from build123d import *

# Parameters (mm, degrees)
FORO_SVASATO_PER_VITE_M5_1_D           = 5
FORO_SVASATO_PER_VITE_M5_1_CSINK_D     = 8.6
FORO_SVASATO_PER_VITE_M5_1_CSINK_ANGLE = 90
RIPETIZIONECIRCOLARE1_COUNT            = 4


with BuildPart() as part:
    # Schizzo1 → Rivoluzione1 (revolve)
    with BuildSketch(Plane.XY, mode=Mode.PRIVATE) as rivoluzione1_sk:
        Polygon((6.5, 0), (6.5, 4), (9, 4), (9, 9), (23, 9), (23, 4.7), (12.5, 4.7), (12.5, 0), align=None)
    revolve(rivoluzione1_sk.sketch.rotate(Axis((0, 0, 0), (0, 1, 0)), 90), axis=Axis((0, 0, 0), (0, 1, 0)))

    # Foro svasato per Vite M5-1 (through all)
    with Locations(Plane(origin=(0, 4.7, 0), x_dir=(-1, 0, 0), z_dir=(0, -1, 0))):
        with Locations((-17.5, 0)):
            foro_svasato_per_vite_m5_1 = CounterSinkHole(FORO_SVASATO_PER_VITE_M5_1_D / 2, FORO_SVASATO_PER_VITE_M5_1_CSINK_D / 2, counter_sink_angle=FORO_SVASATO_PER_VITE_M5_1_CSINK_ANGLE)

    # RipetizioneCircolare1: Foro svasato per Vite M5-1 ×4 about axis
    ripetizionecircolare1_axis = Axis((0, 0, 0), (0, 1, 0))
    for i in range(1, RIPETIZIONECIRCOLARE1_COUNT):
        add(foro_svasato_per_vite_m5_1.rotate(ripetizionecircolare1_axis, i * 360 / RIPETIZIONECIRCOLARE1_COUNT), mode=Mode.SUBTRACT)


solid = part.part
CAD build for the part. Positions are in the model's coordinates, mm. A direction names the side the tool comes from. Give positions to 0.01 mm unless a question says otherwise; leave off trailing zeros. Loops run counter-clockwise (first coordinate to the right, second up) from the corner with the lowest first, then second, coordinate; pieces in that order, holes last. Notation, with made-up numbers: M 74,83.5 L 103,83.5 A20 ccw 103,100.5 Z; hole C -17.75,-35 d7. An arc over 180 degrees is marked long. One line per question, with ' | ' between items. Start each with the question number.
1. 3-axis set-ups, long thin cutter, end or side, ignore diameter. For faces 1 (the face through (10, 4.7, -10)), 2 (the face through (6, 4, 3)), 3 (the face through (15, 8, 0)): which of +Z, -Z, +X, -X, +Y, -Y reach the whole face in a straight line?
2. Saw through at A-A on x = 0. Give the cut face in (y, z), plus the area to 3 significant figures.
3. Saw through at C-C on y = 5.25. Give the cut face in (x, z).
4. Saw through at D-D on z = 0. Give the cut face in (x, y).
5. Two-plate mould, pull along X, no slides. Class faces 4 (the face through (-3.755, 2.317, -11.923)), 5 (the face through (0, 9, 10)), 6 (the face through (-15, 8, 0)): pulls with the +X half, pulls with the -X half, needs draft (parallel to the pull), parting line crosses it, or undercut.
6. Probe L1, parallel to Z at x = 17.5, y = 7.4; L2, parallel to Y at x = -16.5, z = -14. List the from-to ranges inside material, lowest first. Write a range as from..to.
7. Flat gauge pins, fed straight in: pin 1 (14 mm diameter, centred on x = -6.5, z = 7, fed in from -Y); pin 2 (1 mm diameter, centred on y = 6.5, z = 15, fed in from -X); pin 3 (4 mm diameter, centred on y = 7, z = 12, fed in from -X); pin 4 (4.5 mm diameter, centred on x = -17.5, z = 0, fed in from -Y). Where does each tip first touch, or does it go through?
8. Saw through at B-B on z = 17.5. Give the cut face in (x, y).
Result sheet:
1) face 1: -Y | face 2: +Y | face 3: +Y, -Y
2) outline: M 0,-12.5 L 4.7,-12.5 L 4.7,-13.2 L 6.5,-15 L 9,-15 L 9,-9 L 4,-9 L 4,-6.5 L 0,-6.5 Z; M 0,6.5 L 4,6.5 L 4,9 L 9,9 L 9,15 L 6.5,15 L 4.7,13.2 L 4.7,12.5 L 0,12.5 Z; M 4.7,-23 L 9,-23 L 9,-20 L 6.5,-20 L 4.7,-21.8 Z; M 4.7,21.8 L 6.5,20 L 9,20 L 9,23 L 4.7,23 Z | area: 124 mm^2
3) outline: C 0,0 d46; hole C -17.5,0 d7.5; hole C 0,0 d18; hole C 0,-17.5 d7.5; hole C 0,17.5 d7.5; hole C 17.5,0 d7.5
4) outline: M -23,4.7 L -21.8,4.7 L -20,6.5 L -20,9 L -23,9 Z; M -15,6.5 L -13.2,4.7 L -12.5,4.7 L -12.5,0 L -6.5,0 L -6.5,4 L -9,4 L -9,9 L -15,9 Z; M 6.5,0 L 12.5,0 L 12.5,4.7 L 13.2,4.7 L 15,6.5 L 15,9 L 9,9 L 9,4 L 6.5,4 Z; M 20,6.5 L 21.8,4.7 L 23,4.7 L 23,9 L 20,9 Z
5) face 4: parting line crosses it | face 5: needs draft | face 6: undercut
6) L1: z = -14.92..-2.5, 2.5..14.92 | L2: y = 4.7..9
7) pin 1: stops at y = 0 | pin 2: stops at x = -17.85 | pin 3: stops at x = -20.71 | pin 4: passes through
8) outline: M -14.92,4.7 L -4.3,4.7 L -2.5,6.5 L -2.5,9 L -14.92,9 Z; M 2.5,6.5 L 4.3,4.7 L 14.92,4.7 L 14.92,9 L 2.5,9 Z
